Work out the finished part from the listing and answer in its coordinate system (mm). Face numbers are marked on the shaded views. A direction names the side the tool comes from. Round coordinates to 2 decimals unless told otherwise and drop trailing zeros. Loops run counter-clockwise (first coordinate to the right, second up) from the corner with the lowest first, then second, coordinate; pieces in that order, holes last.
from build123d import *

# Parameters (mm, degrees)
EXTRUDE_1_DEPTH = 10
SKETCH_1_6_R    = 2.7
EXTRUDE_2_DEPTH = 8
EXTRUDE_START   = -2
EXTRUDE_3_DEPTH = 2
FILLET_1_R      = 2
FILLET_5_R      = 2
CHAMFER_1_SIZE  = 0.2


with BuildPart() as part:
    # Sketch 1 → Extrude 1 (new body)
    with BuildSketch(Plane.XY):
        with BuildLine():
            ThreePointArc((-15, 13), (-14.414213562, 14.414213562), (-13, 15))
            Line((-13, 15), (13, 15))
            ThreePointArc((13, 15), (14.414213562, 14.414213562), (15, 13))
            Line((15, 13), (15, -13))
            ThreePointArc((15, -13), (14.414213562, -14.414213562), (13, -15))
            Line((13, -15), (-13, -15))
            ThreePointArc((-13, -15), (-14.414213562, -14.414213562), (-15, -13))
            Line((-15, -13), (-15, 13))
        make_face()
        with BuildLine():
            ThreePointArc((-13, -11), (-12.414213562, -12.414213562), (-11, -13))
            Line((-11, -13), (11, -13))
            ThreePointArc((11, -13), (12.414213562, -12.414213562), (13, -11))
            Line((13, -11), (13, 11))
            ThreePointArc((13, 11), (12.414213562, 12.414213562), (11, 13))
            Line((11, 13), (-11, 13))
            ThreePointArc((-11, 13), (-12.414213562, 12.414213562), (-13, 11))
            Line((-13, 11), (-13, -11))
        make_face(mode=Mode.SUBTRACT)
    extrude(amount=EXTRUDE_1_DEPTH)



with BuildPart() as body_2:
    # Sketch 1_6 → Extrude 2 (new body)
    with BuildSketch(Plane.XY):
        Circle(SKETCH_1_6_R)
        Polygon((-2.075, -0.575), (-2.075, 0.575), (-0.575, 0.575), (-0.575, 2.075), (0.575, 2.075), (0.575, 0.575), (2.075, 0.575), (2.075, -0.575), (0.575, -0.575), (0.575, -2.075), (-0.575, -2.075), (-0.575, -0.575), align=None, mode=Mode.SUBTRACT)
    extrude(amount=EXTRUDE_2_DEPTH)


with BuildPart() as part_1:
    add(part.part)

    add(body_2.part)  # Extrude 3 merges body 2
    # Sketch 1_7 → Extrude 3 (add)
    with BuildSketch(Plane.XY.offset(EXTRUDE_START)):
        with BuildLine():
            Line((-13, 15), (13, 15))
            ThreePointArc((13, 15), (14.414213562, 14.414213562), (15, 13))
            Line((15, 13), (15, -13))
            ThreePointArc((15, -13), (14.414213562, -14.414213562), (13, -15))
            Line((13, -15), (-13, -15))
            ThreePointArc((-13, -15), (-14.414213562, -14.414213562), (-15, -13))
            Line((-15, -13), (-15, 13))
            ThreePointArc((-15, 13), (-14.414213562, 14.414213562), (-13, 15))
        make_face()
    extrude(amount=EXTRUDE_3_DEPTH)

    # Fillet 1
    fillet_1_edges = [part_1.edges().sort_by_distance(p)[0] for p in [
        (-14.414213562, -14.414213562, -2),
        (-15, 0, -2),
        (14.414213562, 14.414213562, -2),
        (14.414213562, -14.414213562, -2),
        (0, -15, -2),
        (-14.414213562, 14.414213562, -2),
        (0, 15, -2),
        (15, 0, -2),
    ]]
    fillet(fillet_1_edges, radius=FILLET_1_R)

    # Fillet 5
    fillet_5_edges = [part_1.edges().sort_by_distance(p)[0] for p in [
        (0, -13, 0),
        (12.414213562, -12.414213562, 0),
        (13, 0, 0),
        (12.414213562, 12.414213562, 0),
        (0, 13, 0),
        (-12.414213562, 12.414213562, 0),
        (-13, 0, 0),
        (-12.414213562, -12.414213562, 0),
        (-2.7, 0, 0),
    ]]
    fillet(fillet_5_edges, radius=FILLET_5_R)

    # Chamfer 1
    chamfer_1_edges = [part_1.edges().sort_by_distance(p)[0] for p in [
        (1.325, -0.575, 8),
        (0, -2.075, 8),
        (-0.575, -1.325, 8),
        (-1.325, -0.575, 8),
        (-2.075, 0, 8),
        (-0.575, 1.325, 8),
        (0, 2.075, 8),
        (0.575, 1.325, 8),
        (1.325, 0.575, 8),
        (2.075, 0, 8),
        (0.575, -1.325, 8),
        (-1.325, 0.575, 8),
    ]]
    chamfer(chamfer_1_edges, length=CHAMFER_1_SIZE)


solid = part_1.part
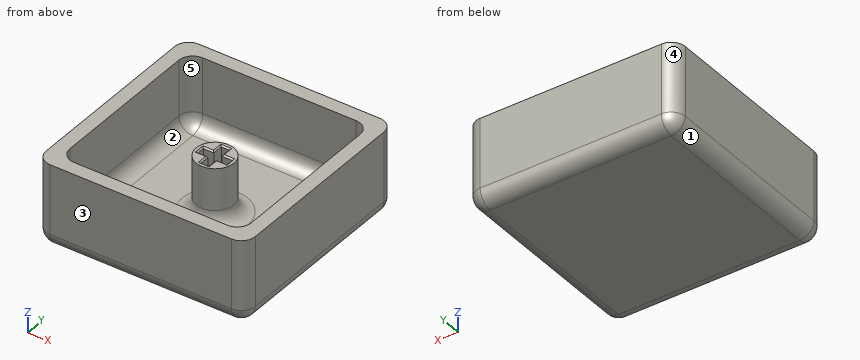
Item 1: Section B-B, the plane x = 0 is taken. Give the vertices of the cut face in (y, z) (3 decimals).
Item 2: Straight lines are drawn through the part: line 1 (X direction, y = -5, z = 3); line 2 (X direction, y = -0.75, z = 0.25) (3 decimals). For each, find the intervals that lie inside material, in ascending order.
Item 3: Section D-D, the plane x = -7 is taken. Give the vertices of the cut face in (y, z).
Item 4: Determine the mould class of the marked faces 1, 2 and 3 for opening direction X: pulls with the +X half, pulls with the -X half, needs draft (parallel to the pull), parting line crosses it, or undercut.
Item 5: Section A-A, the plane z = 2.5 is taken. State how many separate pieces and enclosed holes the cut face has, plus the area to 3 significant figures.
Item 6: For the marked faces 4 and 5, determine the directions among +Z, -Z, +X, -X, +Y, -Y from which every point of the face is accessible in a straight line to the end or side of a thin tool.
Item 7: Each of these flat-tipped pins is pushed along its axis until it touches: P1, Ø4.5, axis at x = 1, y = 0.5, coming from the +Z side; P2, Ø4, axis at x = 8.5, y = 4, coming from the +Z side; P3, Ø12, axis at x = 9, y = 6.5, coming from the +Z side. Where does it stop, or does it pass through?
Answer below:
1. outline: (-15, 0) arc R2 ccw to (-13, -2) - (13, -2) arc R2 ccw to (15, 0) - (15, 10) - (13, 10) - (13, 2) arc R2 cw to (11, 0) - (4.7, 0) arc R2 cw to (2.7, 2) - (2.7, 8) - (2.275, 8) - (2.075, 7.8) - (2.075, 0) - (-2.075, 0) - (-2.075, 7.8) - (-2.275, 8) - (-2.7, 8) - (-2.7, 2) arc R2 cw to (-4.7, 0) - (-11, 0) arc R2 cw to (-13, 2) - (-13, 10) - (-15, 10) - close
2. line 1: x = -15 to -13, 13 to 15
2. line 2: x = -15 to -11.968, -3.656 to -0.575, 0.575 to 3.656, 11.968 to 15
3. outline: (-15, 0) arc R2 ccw to (-13, -2) - (13, -2) arc R2 ccw to (15, 0) - (15, 10) - (13, 10) - (13, 2) arc R2 cw to (11, 0) - (-11, 0) arc R2 cw to (-13, 2) - (-13, 10) - (-15, 10) - close
4. face 1: pulls with the -X half
4. face 2: undercut
4. face 3: needs draft
5. separate pieces: 2
5. enclosed holes: 2
5. area: 239 mm2
6. face 4: +Z, -Z, -X, +Y
6. face 5: +Z
7. P1: stops at z = 8
7. P2: stops at z = 0
7. P3: stops at z = 10
